Verification items for the finished model (mm, model axes). A direction names the side the tool comes from. Coordinates: 2 decimals unless noted, no trailing zeros. Loops run counter-clockwise (first coordinate to the right, second up) from the corner with the lowest first, then second, coordinate; pieces in that order, holes last. Notation, with made-up numbers: (60, 85) -> (70, 85) arc R14 cw to (70, 94) -> close; hole circle Ø11 at (72.25, -2). An arc over 180 degrees is marked (long way). Write item = value, one per line.
```python
from build123d import *

# Parameters (mm, degrees)
SKETCH1_W             = 1.016
SKETCH1_H             = 38.1
BOSS_EXTRUDE2_DEPTH   = 107.95
BOSS_EXTRUDE2_2_DEPTH = 107.95
SKETCH2_W             = 38.1
SKETCH2_H             = 38.1
BOSS_EXTRUDE3_DEPTH   = 83.312
CUT_EXTRUDE1_REACH    = 85.312
SKETCH3_W             = 19.05
SKETCH3_H             = 38.1


with BuildPart() as part:
    # Sketch1 → Boss-Extrude2 (new body, symmetric)
    with BuildSketch(Plane(origin=(0, 0, 0), x_dir=(0, 0, -1), z_dir=(1, 0, 0))):
        with Locations((41.148, 0)):
            Rectangle(SKETCH1_W, SKETCH1_H)
    extrude(amount=BOSS_EXTRUDE2_DEPTH, both=True)



with BuildPart() as body_2:
    # Sketch1 → Boss-Extrude2 2 (new body, symmetric)
    with BuildSketch(Plane(origin=(0, 0, 0), x_dir=(0, 0, -1), z_dir=(1, 0, 0))):
        with Locations((-41.148, 0)):
            Rectangle(SKETCH1_W, SKETCH1_H)
    extrude(amount=BOSS_EXTRUDE2_2_DEPTH, both=True)


with BuildPart() as part_1:
    add(part.part)

    add(body_2.part)  # Boss-Extrude3 merges body 2
    # Sketch2 → Boss-Extrude3 (add)
    with BuildSketch(Plane.XY.offset(41.656)):
        with Locations((127, 0)):
            Rectangle(SKETCH2_W, SKETCH2_H)
    boss_extrude3 = extrude(amount=-BOSS_EXTRUDE3_DEPTH)

    # Mirror4: Boss-Extrude3 across plane
    add(boss_extrude3.mirror(Plane(origin=(0, 0, 0), x_dir=(0, 0, 1), z_dir=(1, 0, 0))))

    # Sketch3 → Cut-Extrude1 (cut, up to next)
    with BuildSketch(Plane(origin=(0, 0, -41.656), x_dir=(-1, 0, 0), z_dir=(0, 0, -1)), mode=Mode.PRIVATE) as cut_extrude1_sk1:
        Rectangle(SKETCH3_W, SKETCH3_H)
    cut_extrude1_tool1 = extrude(cut_extrude1_sk1.sketch, amount=-CUT_EXTRUDE1_REACH, mode=Mode.PRIVATE) & part_1.part
    add(cut_extrude1_tool1.solids().sort_by_distance((0, 0, -41.656))[0], mode=Mode.SUBTRACT)


solid = part_1.part
```
1) Tool access check on faces 1 (the face through (-107.95, 0, 1)), 2 (the face through (146.05, 0, 1)). Record the directions out of +Z, -Z, +X, -X, +Y, -Y that give a thin tool (end or side, any length) a straight path to the whole face; none if there is none.
Ans:
face_1 = +Y, -Y
face_2 = +Z, -Z, +X, +Y, -Y
2) Release check for a two-part mould opening along Z. For faces 3 (the face through (79, 0, -41.656)), 4 (the face through (-58, 0, -40.64)), 5 (the face through (109, 19.05, 3)) record: pulls with the +Z half, pulls with the -Z half, needs draft (parallel to the pull), parting line crosses it, or undercut.
Ans:
face_3 = pulls with the -Z half
face_4 = undercut
face_5 = needs draft
3) Sectioned sample at A-A, the plane z = -32.5. Record the cut outline in (x, y), plus the area to 3 significant figures.
Ans:
outline = (-146.05, -19.05) -> (-107.95, -19.05) -> (-107.95, 19.05) -> (-146.05, 19.05) -> close; (107.95, -19.05) -> (146.05, -19.05) -> (146.05, 19.05) -> (107.95, 19.05) -> close
area = 2,900 mm2
4) Sectioned sample at B-B, the plane x = -95. Record the cut outline in (y, z), plus the area to 3 significant figures.
Ans:
outline = (-19.05, -41.66) -> (19.05, -41.66) -> (19.05, -40.64) -> (-19.05, -40.64) -> close; (-19.05, 40.64) -> (19.05, 40.64) -> (19.05, 41.66) -> (-19.05, 41.66) -> close
area = 77.4 mm2
5) Material ranges on line 1 (X direction, y = 10, z = 24.5); line 2 (Z direction, x = -91.5, y = 3); line 3 (Z direction, x = 2, y = 16), recorded low to high.
Ans:
line_1 = -146.05 to -107.95, 107.95 to 146.05
line_2 = -41.66 to -40.64, 40.64 to 41.66
line_3 = 40.64 to 41.66
